Part model, mm, in its own coordinate system. A direction names the side the tool comes from. Coordinates: 2 decimals unless noted, no trailing zeros. Write each loop counter-clockwise with the first axis right and the second up, starting at its lowest first coordinate (ties: lowest second). Pieces come first, ordered by that corner, then holes. Notation, with made-up numbers: (16, -23) -> (30, -23) arc R7 ccw to (30, -14) -> close; hole circle Ø6 at (69.25, -9.5). An arc over 180 degrees is marked (long way). Write item = value, one per line.
from build123d import *

# Parameters (mm, degrees)
SKETCH1_W           = 8
SKETCH1_H           = 71
BOSS_EXTRUDE1_DEPTH = 12.5
BOSS_EXTRUDE2_DEPTH = 42
CUT_EXTRUDE1_REACH  = 91.61
CHAMFER1_SIZE       = 15
CHAMFER1_SIZE2      = 10.503113073


with BuildPart() as part:
    # Sketch1 → Boss-Extrude1 (new, symmetric)
    with BuildSketch(Plane(origin=(0, 0, 0), x_dir=(0, 0, -1), z_dir=(1, 0, 0))):
        with Locations((-4, 35.5)):
            Rectangle(SKETCH1_W, SKETCH1_H)
    extrude(amount=BOSS_EXTRUDE1_DEPTH, both=True)

    # Sketch1_3 → Boss-Extrude2 (add, symmetric)
    with BuildSketch(Plane(origin=(0, 0, 0), x_dir=(0, 0, -1), z_dir=(1, 0, 0))):
        Polygon((-35, 0), (-8, 0), (-8, 71), (-35, 71), (-35, 47), (-23, 47), (-23, 10), (-35, 10), align=None)
    extrude(amount=BOSS_EXTRUDE2_DEPTH, both=True)

    # Sketch2 → Cut-Extrude1 (cut, up to next)
    with BuildSketch(Plane.XY, mode=Mode.PRIVATE) as cut_extrude1_sk1:
        Polygon((42, 71), (42, 35), (30.310663322, 53), (8.082514505, 71), align=None)
    cut_extrude1_tool1 = extrude(cut_extrude1_sk1.sketch, amount=CUT_EXTRUDE1_REACH, mode=Mode.PRIVATE) & part.part
    # Sketch2 → Cut-Extrude1 (cut, up to next)
    with BuildSketch(Plane.XY, mode=Mode.PRIVATE) as cut_extrude1_sk2:
        Polygon((-8.082514505, 71), (-30.310663322, 53), (-42, 35), (-42, 71), align=None)
    cut_extrude1_tool2 = extrude(cut_extrude1_sk2.sketch, amount=CUT_EXTRUDE1_REACH, mode=Mode.PRIVATE) & part.part
    # Sketch2 → Cut-Extrude1 (cut, up to next)
    with BuildSketch(Plane.XY, mode=Mode.PRIVATE) as cut_extrude1_sk3:
        with BuildLine():
            ThreePointArc((4, 39), (0, 43), (-4, 39))
            Line((-4, 39), (-4, 18))
            ThreePointArc((-4, 18), (0, 14), (4, 18))
            Line((4, 18), (4, 39))
        make_face()
    cut_extrude1_tool3 = extrude(cut_extrude1_sk3.sketch, amount=CUT_EXTRUDE1_REACH, mode=Mode.PRIVATE) & part.part
    add(cut_extrude1_tool1.solids().sort_by_distance((31.410867, 60.103615, 0))[0], mode=Mode.SUBTRACT)
    add(cut_extrude1_tool2.solids().sort_by_distance((-31.410867, 60.103615, 0))[0], mode=Mode.SUBTRACT)
    add(cut_extrude1_tool3.solids().sort_by_distance((0, 28.5, 0))[0], mode=Mode.SUBTRACT)

    # Chamfer1
    chamfer1_edges = [part.edges().sort_by_distance(p)[0] for p in [
        (0, 71, 35),
    ]]
    chamfer1_side = [part.faces().sort_by_distance(p)[0] for p in [
        (0, 71, 17.5),
    ]]
    chamfer(chamfer1_edges, length=CHAMFER1_SIZE, length2=CHAMFER1_SIZE2, reference=chamfer1_side[0])


solid = part.part
Q1. Saw through at A-A on y = 32. Give the cut face in (x, z).
Model answer:
outline = (-42, 8) -> (-12.5, 8) -> (-12.5, 0) -> (-4, 0) -> (-4, 23) -> (-42, 23) -> close; (4, 0) -> (12.5, 0) -> (12.5, 8) -> (42, 8) -> (42, 23) -> (4, 23) -> close
Q2. Saw through at C-C on x = 0. Give the cut face in (y, z).
Model answer:
outline = (0, 0) -> (14, 0) -> (14, 23) -> (10, 23) -> (10, 35) -> (0, 35) -> close; (43, 0) -> (71, 0) -> (71, 20) -> (60.5, 35) -> (47, 35) -> (47, 23) -> (43, 23) -> close
Q3. Probe line 1 (X direction, y = 19.5, z = 16); line 2 (X direction, y = 38.5, z = 4.5); line 3 (Z direction, x = 26, y = 28). List the from-to ranges inside material, lowest first. Write a range as from..to.
Model answer:
line_1 = -42..-4, 4..42
line_2 = -12.5..-4, 4..12.5
line_3 = 8..23
Q4. Saw through at B-B on z = 15. Give the cut face in (x, y), and give its area (3 significant figures).
Model answer:
outline = (-42, 0) -> (42, 0) -> (42, 35) -> (30.31, 53) -> (8.08, 71) -> (-8.08, 71) -> (-30.31, 53) -> (-42, 35) -> close; hole (-4, 18) arc R4 ccw to (4, 18) -> (4, 39) arc R4 ccw to (-4, 39) -> close
area = 4,710 mm²
Q5. Mould opens along Y. For faces 1 (the face through (4, 28, 11)), 2 (the face through (12.5, 34, 4)), 3 (the face through (19.352, 61.874, 17.255)) say: released by +Y, released by -Y, zero draft, split by the parting line, or undercut.
Model answer:
face_1 = undercut
face_2 = zero draft
face_3 = released by +Y
Q6. Which spindle directions (+Z, -Z, +X, -X, +Y, -Y) get a long thin tool onto all of the face, cutting with end or side? Do faces 4 (the face through (-34.77, 46.13, 18.31)), 5 (the face through (-27, 26, 8)), 6 (the face through (0, 43, 11)), 7 (the face through (0, 47, 29)), 8 (the face through (27, 26, 8)). Say none if no direction does.
Model answer:
face_4 = +Z, -Z, -X, +Y
face_5 = -Z, -X, +Y, -Y
face_6 = +Z, -Z
face_7 = +Z, +X, -X
face_8 = -Z, +X, +Y, -Y
Q7. Pin check, flat tips, straight feed: pin 1 (8 mm diameter, centred on y = 61, z = 23, fed in from +X); pin 2 (1.5 mm diameter, centred on y = 60, z = 26.5, fed in from -X); pin 3 (3.5 mm diameter, centred on x = 20, z = 30.5, fed in from +Y). Stop position of each tip, or through.
Model answer:
pin_1 = 25.37
pin_2 = -22.59
pin_3 = 62.77
Q8. Saw through at D-D on z = 24. Give the cut face in (x, y), and give its area (3 significant figures).
Model answer:
outline = (-42, 0) -> (42, 0) -> (42, 10) -> (-42, 10) -> close; (-34.21, 47) -> (34.21, 47) -> (30.31, 53) -> (11.54, 68.2) -> (-11.54, 68.2) -> (-30.31, 53) -> close
area = 1,860 mm²
